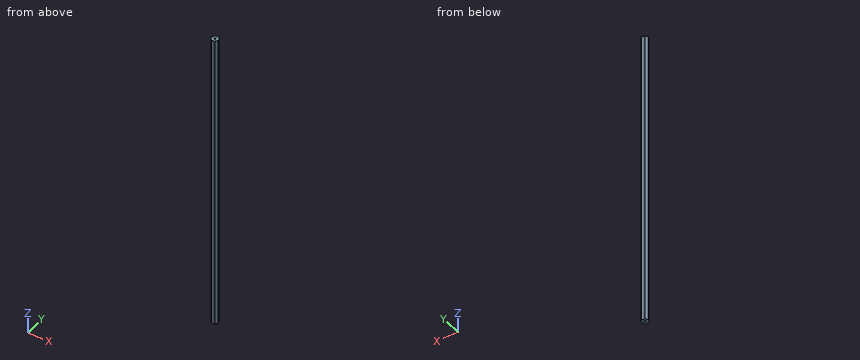
from build123d import *

# Parameters (mm, degrees)
SKETCH1_R           = 2.000000064
BOSS_EXTRUDE1_DEPTH = 609.6


with BuildPart() as part:
    # Sketch1 → Boss-Extrude1 (new body)
    with BuildSketch(Plane.XY):
        with BuildLine():
            ThreePointArc((4.181770846, 5.456960429), (3.437499983, 5.953924622), (2.634980936, 6.35))
            Line((2.634980936, 6.35), (-2.634980936, 6.35))
            ThreePointArc((-2.634980936, 6.35), (-3.437499983, 5.953924622), (-4.181770846, 5.456960429))
            Line((-4.181770846, 5.456960429), (-6.816751782, 0.893039571))
            ThreePointArc((-6.816751782, 0.893039571), (-6.874999966, 0), (-6.816751782, -0.893039571))
            Line((-6.816751782, -0.893039571), (-4.181770846, -5.456960429))
            ThreePointArc((-4.181770846, -5.456960429), (-3.437499983, -5.953924622), (-2.634980936, -6.35))
            Line((-2.634980936, -6.35), (2.634980936, -6.35))
            ThreePointArc((2.634980936, -6.35), (3.437499983, -5.953924622), (4.181770846, -5.456960429))
            Line((4.181770846, -5.456960429), (6.816751782, -0.893039571))
            ThreePointArc((6.816751782, -0.893039571), (6.860422465, -0.447468582), (6.874999966, 0))
            ThreePointArc((6.874999966, 0), (6.860422465, 0.447468582), (6.816751782, 0.893039571))
            Line((6.816751782, 0.893039571), (4.181770846, 5.456960429))
        make_face()
        with Locations(Location((0, 0, 0), (0, 0, 180))):
            Circle(SKETCH1_R, mode=Mode.SUBTRACT)
    extrude(amount=BOSS_EXTRUDE1_DEPTH)


solid = part.part
Model file for the job. Use its own axes, mm. Coordinates: 2 decimals unless noted, no trailing zeros. Write each loop counter-clockwise with the first axis right and the second up, starting at its lowest first coordinate (ties: lowest second). Pieces come first, ordered by that corner, then holes. Notation, with made-up numbers: (-9, 30) - (4, 30) arc R20 ccw to (4, 61) - close; hole circle Ø5 at (-8, 47). An arc over 180 degrees is marked (long way). Write each question's results on one line, items separated by ' | '. Start each with the question number.
1) Cut at A-A (z = 530.5). Write the cut outline in (x, y) (3 decimals), then the cut area to 3 significant figures.
2) Flat gauge pins, fed straight in: P1, Ø3, axis at x = 0, y = 0, coming from the +Z side; P2, Ø1, axis at y = 4.5, z = 268.5, coming from the +X side; P3, Ø3, axis at y = -3.5, z = 338, coming from the -X side; P4, Ø3, axis at y = 5, z = 398, coming from the +X side. Where does each tip first touch, or does it go through?
3) Probe line 1 along Y through (x, z) = (-0.5, 295); line 2 along Y through (x, z) = (0, 252); line 3 along X through (y, z) = (-0.5, 496). List the from-to ranges inside material, lowest first. Write a range as from..to.
Returned:
1) outline: (-6.817, -0.893) - (-4.182, -5.457) arc R6.875 ccw to (-2.635, -6.35) - (2.635, -6.35) arc R6.875 ccw to (4.182, -5.457) - (6.817, -0.893) arc R6.875 ccw to (6.817, 0.893) - (4.182, 5.457) arc R6.875 ccw to (2.635, 6.35) - (-2.635, 6.35) arc R6.875 ccw to (-4.182, 5.457) - (-6.817, 0.893) arc R6.875 ccw to start; hole circle Ø4 at (0, 0) | area: 125 mm^2
2) P1: through | P2: x = 5.02 | P3: x = -6.18 | P4: x = 5.31
3) line 1: -6.35..-1.94, 1.94..6.35 | line 2: -6.35..-2, 2..6.35 | line 3: -6.86..-1.94, 1.94..6.86
